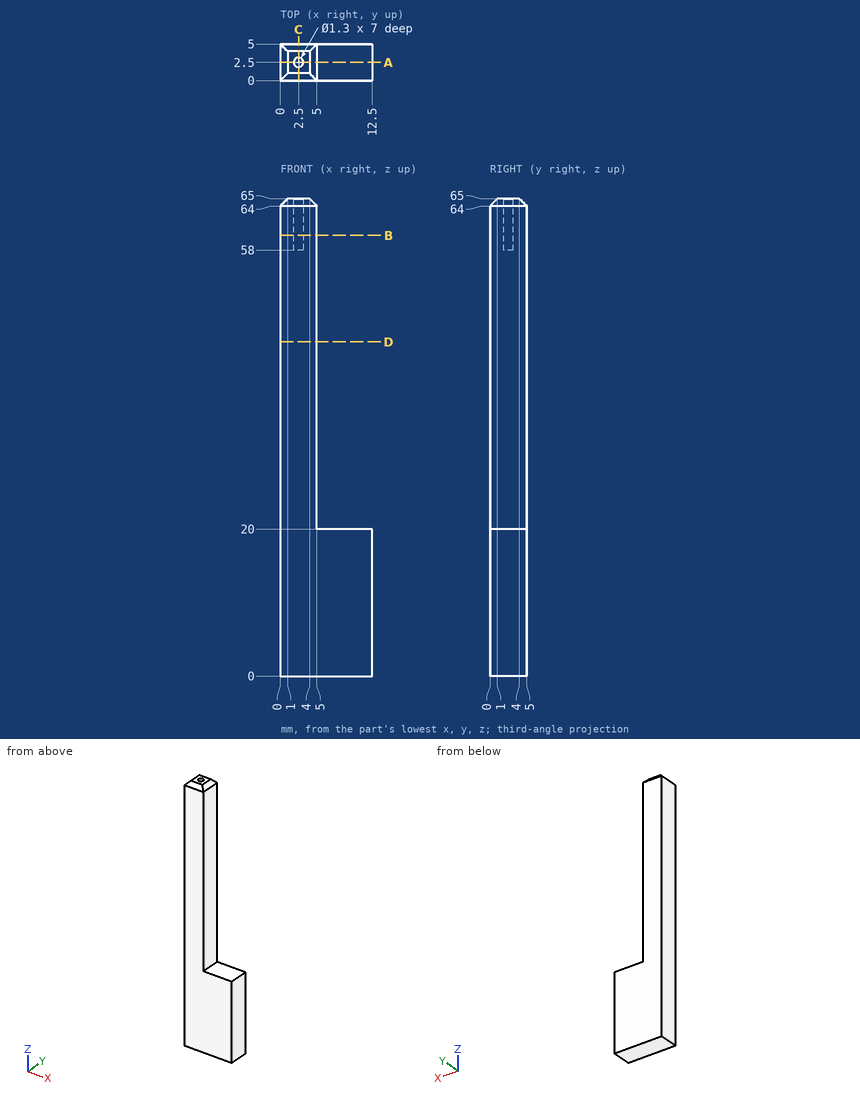
Source: three-view drawing plus pictorial views. Frame: mm from the lowest corner of the part. Round coordinates to 2 decimals unless told otherwise and drop trailing zeros. Write each loop counter-clockwise with the first axis right and the second up, starting at its lowest first coordinate (ties: lowest second). Pieces come first, ordered by that corner, then holes. Notation, with made-up numbers: M -25.5,73 L -15.5,73 A11 ccw -15.5,87 Z; hole C -10.5,-34.5 d4. An arc over 180 degrees is marked long. Use CSV: the item, a comma, the result in double quotes. Start each with the question number.
Q1. Line query: line 1 (Y direction, x = 2.5, z = 63); line 2 (X direction, y = 4.8, z = 32); line 3 (Z direction, x = 10, y = 4.05). Output: solid intervals per line, ascending. Write a range as from..to.
Q2. Cut plane A-A on y = 2.5. Output: boundary loops of the cut face in (x, z).
Q3. Cut plane D-D on z = 45.5. Output: boundary loops of the cut face in (x, y), plus the area to 3 significant figures.
Q4. Cut plane C-C on x = 2.5. Output: boundary loops of the cut face in (y, z), plus the area to 3 significant figures.
Q5. Cut plane B-B on z = 60. Output: boundary loops of the cut face in (x, y).
Q6. First-contact query: P1, Ø2.5, axis at x = 9, y = 2.5, coming from the +Z side; P2, Ø3, axis at x = 6, y = 3, coming from the +Z side. Flat tips, straight axial feed; report the tip coordinate or a pass-through.
Results found:
1,line 1,"0..1.85, 3.15..5"
1,line 2,"0..5"
1,line 3,"0..20"
2,outline,"M 0,0 L 12.5,0 L 12.5,20 L 5,20 L 5,64 L 4,65 L 3.15,65 L 3.15,58 L 1.85,58 L 1.85,65 L 1,65 L 0,64 Z"
3,outline,"M 0,0 L 5,0 L 5,5 L 0,5 Z"
3,area,"25.0 mm^2"
4,outline,"M 0,0 L 5,0 L 5,64 L 4,65 L 3.15,65 L 3.15,58 L 1.85,58 L 1.85,65 L 1,65 L 0,64 Z"
4,area,"315 mm^2"
5,outline,"M 0,0 L 5,0 L 5,5 L 0,5 Z; hole C 2.5,2.5 d1.3"
6,P1,"z = 20"
6,P2,"z = 64.5"
